Can you work these out from the model? Positions are in its coordinate system, mm. Face numbers are marked on the shaded views. A direction names the side the tool comes from. Round coordinates to 2 decimals unless told otherwise and drop trailing zeros. Write each loop counter-clockwise with the first axis right and the second up, starting at its lowest first coordinate (ties: lowest second). Pieces come first, ordered by that corner, then holes. Notation, with made-up numbers: M 67,-21 L 72,-21 A20 cw 72,15 Z; hole C 63,50.25 d6. An arc over 180 degrees is marked long. Answer as a JSON object with one key per item and string values. Group by question number.
1) Suppose I cut it at A-A, the plane x = -11.5. Write out the boundary of the cut face in (y, z).
2) On a 3-axis mill with a long thin cutter (end or side, diameter ignored), from which of +Z, -Z, +X, -X, +Y, -Y can I reach the whole of each face in a straight line? I mean the marked faces 5, 6 and 7. Say none if no direction works.
3) Suppose I cut it at C-C, the plane y = -3. Write out the boundary of the cut face in (x, z), and give its area (3 significant figures).
4) Please list where these lines run through material, in increasing order: L1, parallel to Z at x = -31.5, y = -2; L2, parallel to Z at x = -40, y = -4.75; L3, parallel to Z at x = -7, y = -6.75. Write a range as [from, to].
5) I'm going to push flat-ended pins straight in: pin 1 Ø5 at (x, y) = (-11.5, -16) entering from -Z; pin 2 Ø1.5 at (y, z) = (-13.5, -6.5) entering from +X; pin 3 Ø2 at (x, y) = (-28, -4.5) entering from +Z. Where does each tip first touch, or does it pass through?
6) Suppose I cut it at B-B, the plane z = -11. Write out the boundary of the cut face in (x, y), and give its area (3 significant figures).
7) Suppose I cut it at D-D, the plane z = 0. Write out the boundary of the cut face in (x, y).
8) If we mould it in two halves opening along Z, with no side actions, what happens to the marked faces 1, 2, 3 and 4? For each: +Z half, -Z half, draft (parallel to the pull), parting line (faces both ways), or undercut.
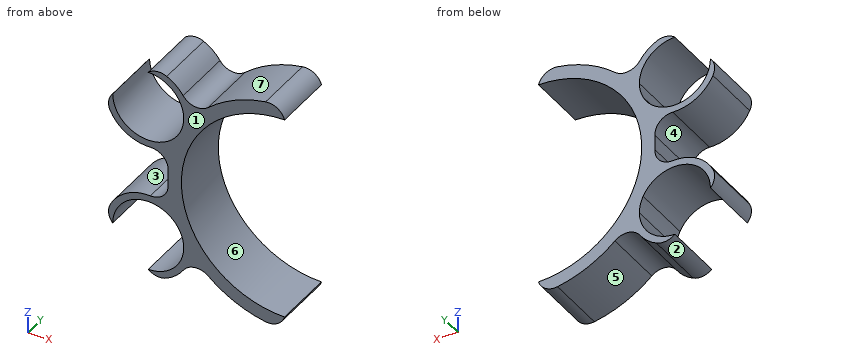
from build123d import *

# Parameters (mm, degrees)
F1_DEPTH     = 18
F2_T1_DEPTH  = 18
F2_T3_DEPTH  = 18
F2_T5_DEPTH  = 18
F2_T7_DEPTH  = 18
F2_T9_DEPTH  = 46.171808491
F2_T11_DEPTH = 46.171808491
F2_T13_DEPTH = 46.171808491
F2_T15_DEPTH = 46.171808491
F2_T17_DEPTH = 46.1730452367
F2_T19_DEPTH = 46.1730452367


# Not quite as in the source:
# - a fillet or chamfer that OpenCascade refuses, or shapes differently, is made with other operations: its cross-section is extruded or revolved along the edge and cut away or added


with BuildPart() as f1:
    # F0 (on Front) → F1 (new body)
    with BuildSketch(Plane.XZ):
        with BuildLine():
            ThreePointArc((-30.9053214059, 15.3333332579), (-29.4709612635, 17.9363441706), (-27.8178919283, 20.4062463149))
            ThreePointArc((-27.8178919283, 20.4062463149), (-31.6172700774, 28.9813161323), (-40.3112887415, 32.5))
            Line((-40.3112887415, 32.5), (-40.3112887415, 30.5))
            ThreePointArc((-40.3112887415, 30.5), (-32.886667539, 27.4246212025), (-29.8112887415, 20))
            ThreePointArc((-29.8112887415, 20), (-30.0884550584, 17.6034041876), (-30.9053214059, 15.3333332579))
        make_face()
        with BuildLine():
            ThreePointArc((0, -30.5), (-30.5, 0), (0, 30.5))
            Line((0, 30.5), (0, 34.5))
            ThreePointArc((0, 34.5), (-15.5922176443, 30.7755219116), (-27.8178919283, 20.4062463149))
            ThreePointArc((-27.8178919283, 20.4062463149), (-27.8129396472, 20.203149988), (-27.8112887415, 20))
            ThreePointArc((-27.8112887415, 20), (-29.205476311, 14.2631951176), (-33.0770375829, 9.8060993641))
            ThreePointArc((-33.0770375829, 9.8060993641), (-34.5, 0), (-33.0770375829, -9.8060993641))
            ThreePointArc((-33.0770375829, -9.8060993641), (-29.205476311, -14.2631951176), (-27.8112887415, -20))
            ThreePointArc((-27.8112887415, -20), (-27.8129396472, -20.203149988), (-27.8178919283, -20.4062463149))
            ThreePointArc((-27.8178919283, -20.4062463149), (-15.5922176443, -30.7755219116), (0, -34.5))
            Line((0, -34.5), (0, -30.5))
        make_face()
        with BuildLine():
            ThreePointArc((-27.8112887415, 20), (-27.8129396472, 20.203149988), (-27.8178919283, 20.4062463149))
            ThreePointArc((-27.8178919283, 20.4062463149), (-29.4709612635, 17.9363441706), (-30.9053214059, 15.3333332579))
            ThreePointArc((-30.9053214059, 15.3333332579), (-32.1103276855, 12.6165310576), (-33.0770375829, 9.8060993641))
            ThreePointArc((-33.0770375829, 9.8060993641), (-29.205476311, 14.2631951176), (-27.8112887415, 20))
        make_face()
        with BuildLine():
            ThreePointArc((-30.905321409, -15.3333332517), (-29.4709612653, -17.9363441676), (-27.8178919283, -20.4062463149))
            ThreePointArc((-27.8178919283, -20.4062463149), (-27.8129396472, -20.203149988), (-27.8112887415, -20))
            ThreePointArc((-27.8112887415, -20), (-29.205476311, -14.2631951176), (-33.0770375829, -9.8060993641))
            ThreePointArc((-33.0770375829, -9.8060993641), (-32.1103276868, -12.6165310544), (-30.905321409, -15.3333332517))
        make_face()
        with BuildLine():
            ThreePointArc((-33.0770375829, 9.8060993641), (-32.1103276855, 12.6165310576), (-30.9053214059, 15.3333332579))
            ThreePointArc((-30.9053214059, 15.3333332579), (-42.7078845539, 9.7771663169), (-50.8112887415, 20))
            Line((-50.8112887415, 20), (-52.8112887415, 20))
            ThreePointArc((-52.8112887415, 20), (-46.0480936239, 8.8941875695), (-33.0770375829, 9.8060993641))
        make_face()
        with BuildLine():
            ThreePointArc((-50.8112887415, -20), (-42.7078845573, -9.7771663177), (-30.905321409, -15.3333332517))
            ThreePointArc((-30.905321409, -15.3333332517), (-32.1103276868, -12.6165310544), (-33.0770375829, -9.8060993641))
            ThreePointArc((-33.0770375829, -9.8060993641), (-46.0480936239, -8.8941875695), (-52.8112887415, -20))
            Line((-52.8112887415, -20), (-50.8112887415, -20))
        make_face()
        with BuildLine():
            ThreePointArc((-40.3112887415, -32.5), (-31.6172700774, -28.9813161323), (-27.8178919283, -20.4062463149))
            ThreePointArc((-27.8178919283, -20.4062463149), (-29.4709612653, -17.9363441676), (-30.905321409, -15.3333332517))
            ThreePointArc((-30.905321409, -15.3333332517), (-30.0884550592, -17.6034041842), (-29.8112887415, -20))
            ThreePointArc((-29.8112887415, -20), (-32.886667539, -27.4246212025), (-40.3112887415, -30.5))
            Line((-40.3112887415, -30.5), (-40.3112887415, -32.5))
        make_face()
    extrude(amount=F1_DEPTH)

    # F2: fillet of radius 5 on 10 edges, made by hand

    # F2_s2 → F2_t1 (join)
    with BuildSketch(Plane.XZ):
        with BuildLine():
            ThreePointArc((-29.9854181156, 27.0446004725), (-26.4995189962, 24.9041460638), (-22.5822762114, 26.0823848816))
            ThreePointArc((-22.5822762114, 26.0823848816), (-25.3593942038, 23.3912617363), (-27.8178919283, 20.4062463149))
            ThreePointArc((-27.8178919283, 20.4062463149), (-28.4286678987, 23.8798610678), (-29.9854181156, 27.0446004725))
        make_face()
    extrude(amount=F2_T1_DEPTH)

    # F2_s4 → F2_t3 (join)
    with BuildSketch(Plane.XZ):
        with BuildLine():
            ThreePointArc((-39.6741951276, 7.5162460883), (-35.861056634, 6.0353637247), (-34.4295655704, 2.2034097738))
            ThreePointArc((-34.4295655704, 2.2034097738), (-33.9666835234, 6.0427154842), (-33.0770375829, 9.8060993641))
            ThreePointArc((-33.0770375829, 9.8060993641), (-36.2124627952, 8.1911208888), (-39.6741951276, 7.5162460883))
        make_face()
    extrude(amount=F2_T3_DEPTH)

    # F2_s6 → F2_t5 (join)
    with BuildSketch(Plane.XZ):
        with BuildLine():
            ThreePointArc((-34.4295655704, -2.2034097738), (-35.861056634, -6.0353637247), (-39.6741951276, -7.5162460883))
            ThreePointArc((-39.6741951276, -7.5162460883), (-36.2124627952, -8.1911208888), (-33.0770375829, -9.8060993641))
            ThreePointArc((-33.0770375829, -9.8060993641), (-33.9666835234, -6.0427154842), (-34.4295655704, -2.2034097738))
        make_face()
    extrude(amount=F2_T5_DEPTH)

    # F2_s8 → F2_t7 (join)
    with BuildSketch(Plane.XZ):
        with BuildLine():
            ThreePointArc((-29.9854181156, -27.0446004725), (-26.4995189962, -24.9041460638), (-22.5822762114, -26.0823848816))
            ThreePointArc((-22.5822762114, -26.0823848816), (-25.3593942038, -23.3912617363), (-27.8178919283, -20.4062463149))
            ThreePointArc((-27.8178919283, -20.4062463149), (-28.4286678987, -23.8798610678), (-29.9854181156, -27.0446004725))
        make_face()
    extrude(amount=F2_T7_DEPTH)

    # F2_s10 → F2_t9 (cut)
    with BuildSketch(Plane.XZ.offset(-14.0859042455)):
        with BuildLine():
            ThreePointArc((-34.8218866889, 31.2301587302), (-37.676903372, 31.6944428559), (-40.3112887415, 30.5))
            Line((-40.3112887415, 30.5), (-40.3112887415, 32.5))
            ThreePointArc((-40.3112887415, 32.5), (-37.4941078924, 32.1784026893), (-34.8218866889, 31.2301587302))
        make_face()
    extrude(amount=F2_T9_DEPTH, mode=Mode.SUBTRACT)

    # F2_s12 → F2_t11 (cut)
    with BuildSketch(Plane.XZ.offset(-14.0859042455)):
        with BuildLine():
            ThreePointArc((-51.5414474717, 14.5105979474), (-52.0057315974, 17.3656146306), (-50.8112887415, 20))
            Line((-50.8112887415, 20), (-52.8112887415, 20))
            ThreePointArc((-52.8112887415, 20), (-52.4896914308, 17.1828191509), (-51.5414474717, 14.5105979474))
        make_face()
    extrude(amount=F2_T11_DEPTH, mode=Mode.SUBTRACT)

    # F2_s14 → F2_t13 (cut)
    with BuildSketch(Plane.XZ.offset(-14.0859042455)):
        with BuildLine():
            ThreePointArc((-50.8112887415, -20), (-52.0057315974, -17.3656146306), (-51.5414474717, -14.5105979474))
            ThreePointArc((-51.5414474717, -14.5105979474), (-52.4896914308, -17.1828191509), (-52.8112887415, -20))
            Line((-52.8112887415, -20), (-50.8112887415, -20))
        make_face()
    extrude(amount=F2_T13_DEPTH, mode=Mode.SUBTRACT)

    # F2_s16 → F2_t15 (cut)
    with BuildSketch(Plane.XZ.offset(-14.0859042455)):
        with BuildLine():
            ThreePointArc((-34.8218866889, -31.2301587302), (-37.676903372, -31.6944428559), (-40.3112887415, -30.5))
            Line((-40.3112887415, -30.5), (-40.3112887415, -32.5))
            ThreePointArc((-40.3112887415, -32.5), (-37.4941078924, -32.1784026893), (-34.8218866889, -31.2301587302))
        make_face()
    extrude(amount=F2_T15_DEPTH, mode=Mode.SUBTRACT)

    # F2_s18 → F2_t17 (cut)
    with BuildSketch(Plane.XZ.offset(-14.0865226184)):
        with BuildLine():
            ThreePointArc((0, -30.5), (-2.1356819659, -33.3363611882), (-5.6157903729, -34.0398721867))
            ThreePointArc((-5.6157903729, -34.0398721867), (-2.8173045237, -34.3847756314), (0, -34.5))
            Line((0, -34.5), (0, -30.5))
        make_face()
    extrude(amount=F2_T17_DEPTH, mode=Mode.SUBTRACT)

    # F2_s20 → F2_t19 (cut)
    with BuildSketch(Plane.XZ.offset(-14.0865226184)):
        with BuildLine():
            ThreePointArc((-5.6157903729, 34.0398721867), (-2.1356819659, 33.3363611882), (0, 30.5))
            Line((0, 30.5), (0, 34.5))
            ThreePointArc((0, 34.5), (-2.8173045237, 34.3847756314), (-5.6157903729, 34.0398721867))
        make_face()
    extrude(amount=F2_T19_DEPTH, mode=Mode.SUBTRACT)


solid = f1.part
Results:
{
 "1": {"outline": "M -18,-32.53 L 0,-32.53 L 0,-28.25 L -18,-28.25 Z; M -18,28.25 L 0,28.25 L 0,32.53 L -18,32.53 Z"},
 "2": {"face 5": "-Z, +Y, -Y", "face 6": "+X, +Y, -Y", "face 7": "+Z, +Y, -Y"},
 "3": {"outline": "M -51.54,-14.51 A5 ccw -50.81,-20 A10.5 cw long -40.31,-30.5 A5 ccw -34.82,-31.23 A12.5 ccw -29.99,-27.04 A5 cw -22.58,-26.08 A34.5 ccw -5.62,-34.04 A5 ccw 0,-30.5 A30.5 cw 0,30.5 A5 ccw -5.62,34.04 A34.5 ccw -22.58,26.08 A5 cw -29.99,27.04 A12.5 ccw -34.82,31.23 A5 ccw -40.31,30.5 A10.5 cw long -50.81,20 A5 ccw -51.54,14.51 A12.5 ccw -39.67,7.52 A5 cw -34.43,2.2 A34.5 ccw -34.43,-2.2 A5 cw -39.67,-7.52 A12.5 ccw Z", "area": "613 mm^2"},
 "4": {"L1": "[-28.87, -25.71], [-14.29, 14.29], [25.71, 28.87]", "L2": "[-30.75, -30.5], [-9.5, -7.5], [7.5, 9.5], [30.5, 30.75]", "L3": "[-33.78, -29.69], [29.69, 33.78]"},
 "5": {"pin 1": "z = -33.31", "pin 2": "x = -29.63", "pin 3": "z = 25.98"},
 "6": {"outline": "M -48.99,-18 L -45.72,-18 L -45.72,0 L -48.99,0 Z; M -34.9,-18 L -28.45,-18 L -28.45,0 L -34.9,0 Z", "area": "175 mm^2"},
 "7": {"outline": "M -34.5,-18 L -30.5,-18 L -30.5,0 L -34.5,0 Z"},
 "8": {"face 1": "draft", "face 2": "-Z half", "face 3": "undercut", "face 4": "undercut"}
}
